```python
from build123d import *

# Parameters (mm, degrees)
F2_R      = 10.4775
F2_R_2    = 9.2075
F3_DEPTH  = 25.4
F4_DEPTH  = 25.4
F5_W      = 41.5304042399
F5_H      = 20.5683773383
F6_DEPTH  = 127
F7_W      = 46.6519938795
F7_H      = 46.355
F8_DEPTH  = 2.54
F9_W      = 2.54
F9_H      = 46.355
F10_DEPTH = 8.89
F11_W     = 46.6519938795
F11_H     = 46.355
F12_DEPTH = 2.54
F13_R     = 1.7499965
F14_DEPTH = 2.54


with BuildPart() as f3:
    # F2 (on line) → F3 (new body)
    with BuildSketch(Plane(origin=(0, 0, 0), x_dir=(0.9860251287, 0, 0.1665966554), z_dir=(0.1665966554, 0, -0.9860251287))):
        with Locations((41.0343617785, 0)):
            Circle(F2_R)
        with Locations((41.0343617785, 0)):
            Circle(F2_R_2, mode=Mode.SUBTRACT)
    extrude(amount=-F3_DEPTH)

    # F4 (add): a face of the model
    f4_faces = [f3.faces().sort_by_distance(p)[0] for p in [
        (30.422040588, 0, 5.1400416329),
    ]]
    extrude(f4_faces, amount=F4_DEPTH)

    # F5 (on Front) → F6 (cut, symmetric)
    with BuildSketch(Plane.XZ):
        with Locations((39.1329098493, -10.2841886692)):
            Rectangle(F5_W, F5_H)
    extrude(amount=F6_DEPTH, both=True, mode=Mode.SUBTRACT)

    # F7 (on Top) → F8 (join)
    with BuildSketch(Plane.XY):
        with Locations((41.6159391729, 0)):
            Rectangle(F7_W, F7_H)
    extrude(amount=-F8_DEPTH)

    # F9 (on face) → F10 (join)
    with BuildSketch(Plane(origin=(0, 0, -2.54), x_dir=(1, 0, 0), z_dir=(0, 0, -1))):
        with Locations((63.6719361126, 0)):
            Rectangle(F9_W, F9_H)
    extrude(amount=F10_DEPTH)

    # F11 (on face) → F12 (join)
    with BuildSketch(Plane(origin=(0, 0, -11.43), x_dir=(1, 0, 0), z_dir=(0, 0, -1))):
        with Locations((41.6159391729, 0)):
            Rectangle(F11_W, F11_H)
    extrude(amount=F12_DEPTH)

    # F13 (on face) → F14 (cut)
    with BuildSketch(Plane(origin=(0, 0, -13.97), x_dir=(1, 0, 0), z_dir=(0, 0, -1))):
        with Locations((23.9529660876, 0)):
            Circle(F13_R)
        with Locations((56.1965306676, 0)):
            Circle(F13_R)
    extrude(amount=-F14_DEPTH, mode=Mode.SUBTRACT)


solid = f3.part
```
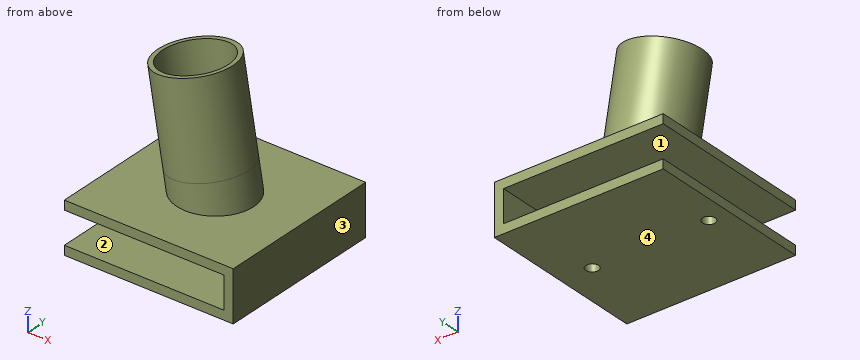
Source: CAD feature listing. Evaluate the final solid. Frame: model axes, mm. Face numbers are marked on the shaded views. Give positions to 0.01 mm unless a question says otherwise; leave off trailing zeros. Order: outer loops, then holes, each group sorted by start corner. A loop starts at its lowest first (then second) coordinate and runs counter-clockwise, first axis right, second up.
(1) Pull-direction query (Z, two-part tool) for the marked faces 1, 2, 3 and 4; classes: +Z half, -Z half, draft (parallel to the pull), parting line (faces both ways), or undercut.
(2) Contact query for flat-ended pins moving along their axis: P1, Ø2, axis at x = 24, z = 26, coming from the +Y side; P2, Ø8, axis at y = -3, z = 15.5, coming from the -X side; P3, Ø8, axis at x = 35, z = 11, coming from the +Y side; P4, Ø4, axis at x = 23.95, y = 0, coming from the +Z side. Output: stop coordinate, or through.
(3) Section query C-C (x = 55.5). Return the cut outline in (y, z).
(4) Material intervals for line 1 along X through (y, z) = (0, -12.8); line 2 along Z through (x, y) = (22, 14.5); line 3 along Y through (x, z) = (35.5, 23.5), sorted ascending.
(5) Section query A-A (x = 61). Return the cut outline in (y, z), plus the area to 3 significant figures.
(6) Section query D-D (y = -20). Return the cut outline in (x, z).
(7) Section query B-B (y = 0). Return the cut outline in (x, z).
Outcome:
1. face 1: undercut
1. face 2: undercut
1. face 3: draft
1. face 4: -Z half
2. P1: passes through
2. P2: stops at x = 27.83
2. P3: stops at y = 10.45
2. P4: stops at z = 30.14
3. outline: (-23.18, -13.97) - (-1.61, -13.97) - (-1.61, -11.43) - (-23.18, -11.43) - close; (-23.18, -2.54) - (23.18, -2.54) - (23.18, 0) - (-23.18, 0) - close; (1.61, -13.97) - (23.18, -13.97) - (23.18, -11.43) - (1.61, -11.43) - close
4. line 1: x = 18.29 to 22.2, 25.7 to 54.45, 57.95 to 64.94
4. line 2: z = -13.97 to -11.43, -2.54 to 0
4. line 3: y = -10.26 to -8.96, 8.96 to 10.26
5. outline: (-23.18, -13.97) - (23.18, -13.97) - (23.18, -11.43) - (-23.18, -11.43) - close; (-23.18, -2.54) - (23.18, -2.54) - (23.18, 0) - (-23.18, 0) - close
5. area: 235 mm2
6. outline: (18.29, -13.97) - (64.94, -13.97) - (64.94, 0) - (18.29, 0) - (18.29, -2.54) - (62.4, -2.54) - (62.4, -11.43) - (18.29, -11.43) - close
7. outline: (18.29, -13.97) - (22.2, -13.97) - (22.2, -11.43) - (18.29, -11.43) - close; (18.29, -2.54) - (62.4, -2.54) - (62.4, -11.43) - (57.95, -11.43) - (57.95, -13.97) - (64.94, -13.97) - (64.94, 0) - (52.24, 0) - (46.56, 33.63) - (45.31, 33.42) - (50.95, 0) - (32.28, 0) - (27.15, 30.35) - (25.9, 30.14) - (30.99, 0) - (18.29, 0) - close; (25.7, -13.97) - (54.45, -13.97) - (54.45, -11.43) - (25.7, -11.43) - close
